Can you work these out from the drawing? Everything is in mm from the part's minimum corner. A direction names the side the tool comes from. Round coordinates to 2 decimals unless told otherwise and drop trailing zeros. Write each loop counter-clockwise with the first axis right and the second up, starting at its lowest first coordinate (ties: lowest second). Pieces come first, ordered by that corner, then holes. Notation, with made-up numbers: (-27, -36) - (30, -36) arc R17 ccw to (30, -17) - close; hole circle Ø3 at (26.25, 50). An arc over 180 degrees is marked (long way). One line per item, written item: value. Start each with the question number.
(1) I want a section at A-A on z = 6.75. List the corners of the cut face in (x, y) for me.
(2) I want a section at D-D on y = 8. List the corners of the cut face in (x, z) for me.
(3) I want a section at B-B on z = 4. List the corners of the cut face in (x, y) for me.
(4) If I drill on L1, parallel to Y at x = 3.25, z = 4; L2, parallel to X at y = 3.25, z = 4; L3, parallel to X at y = 8.5, z = 11.75, over which ranges is the centre line in solid material (lowest first)? Write a range as from..to.
(5) I'm going to push flat-ended pins straight in: pin 1 Ø0.9 at (x, z) = (39, 1.5) entering from +Y; pin 2 Ø5 at (x, z) = (20.5, 15.5) entering from -Y; pin 3 Ø3 at (y, z) = (14.5, 9) entering from -X; pin 4 Ø2 at (x, y) = (47.25, 35.25) entering from -Z. Where does each tip first touch, or does it pass through?
(6) On a 3-axis mill with a long thin cutter (end or side, diameter ignored), from which of +Z, -Z, +X, -X, +Y, -Y can I reach the whole of each face in a straight line? I mean the marked faces 5, 6, 7, 8 and 9. Say none if no direction works.
(7) I want a section at C-C on z = 17. List the corners of the cut face in (x, y) for me, plus the area to 3 significant figures.
(8) Thinking about a two-plate mould opening in X: for the marked faces 1, 2, 3 and 4, which applies, +X half, -X half, draft (parallel to the pull), parting line (faces both ways), or undercut?
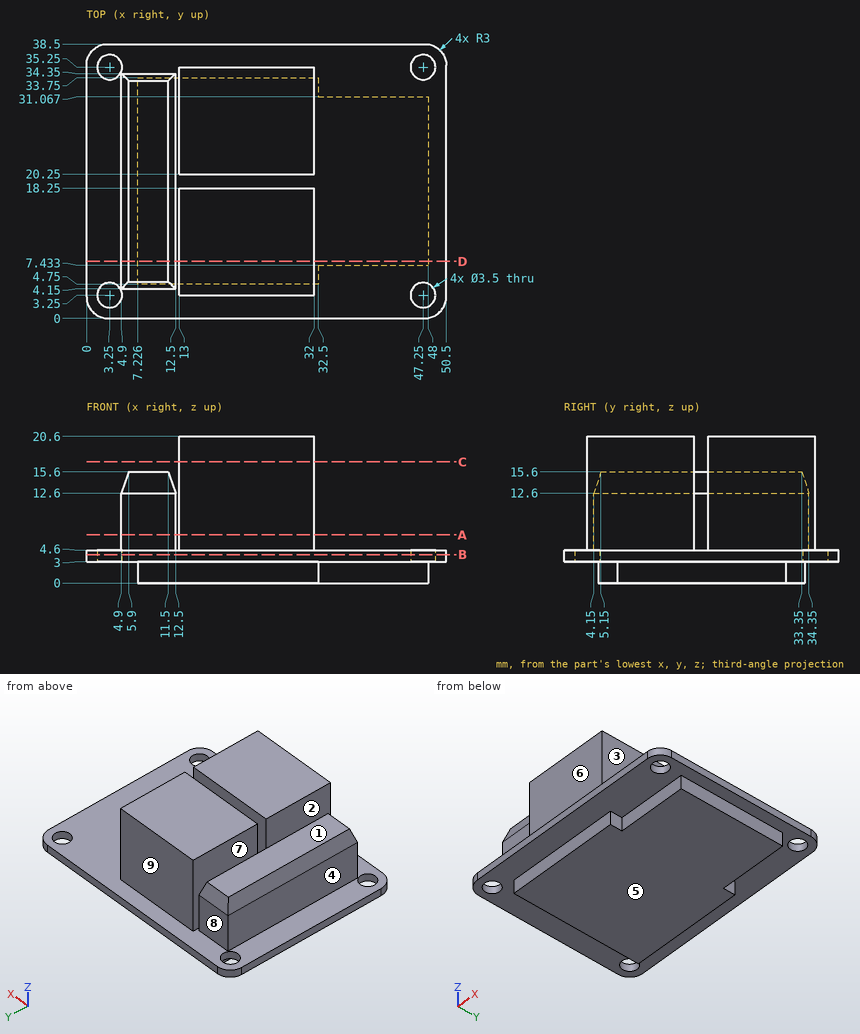
Established:
1. outline: (4.9, 4.15) - (12.5, 4.15) - (12.5, 34.35) - (4.9, 34.35) - close; (13, 3.25) - (32, 3.25) - (32, 18.25) - (13, 18.25) - close; (13, 20.25) - (32, 20.25) - (32, 35.25) - (13, 35.25) - close
2. outline: (0, 3) - (7.23, 3) - (7.23, 0) - (48, 0) - (48, 3) - (50.5, 3) - (50.5, 4.6) - (32, 4.6) - (32, 20.6) - (13, 20.6) - (13, 4.6) - (12.5, 4.6) - (12.5, 12.6) - (11.5, 15.6) - (5.9, 15.6) - (4.9, 12.6) - (4.9, 4.6) - (0, 4.6) - close
3. outline: (0, 3) arc R3 ccw to (3, 0) - (47.5, 0) arc R3 ccw to (50.5, 3) - (50.5, 35.5) arc R3 ccw to (47.5, 38.5) - (3, 38.5) arc R3 ccw to (0, 35.5) - close; hole circle Ø3.5 at (3.25, 3.25); hole circle Ø3.5 at (3.25, 35.25); hole circle Ø3.5 at (47.25, 3.25); hole circle Ø3.5 at (47.25, 35.25)
4. L1: 0..1.5, 5..33.5, 37..38.5
4. L2: 0..1.5, 5..45.5, 49..50.5
4. L3: 4.9..12.5, 13..32
5. pin 1: y = 31.07
5. pin 2: y = 3.25
5. pin 3: x = 4.9
5. pin 4: through
6. face 5: -Z, +X, -X, +Y, -Y
6. face 6: +Z, +X, -X, -Y
6. face 7: +Z, +Y, -Y
6. face 8: +Z, -X, +Y
6. face 9: +Z, +X, -X, +Y
7. outline: (13, 3.25) - (32, 3.25) - (32, 18.25) - (13, 18.25) - close; (13, 20.25) - (32, 20.25) - (32, 35.25) - (13, 35.25) - close
7. area: 570 mm2
8. face 1: draft
8. face 2: undercut
8. face 3: +X half
8. face 4: -X half
